The listing builds one solid part. Answer for the finished solid, in the listing's coordinates (mm). Round coordinates to 2 decimals unless told otherwise and drop trailing zeros. Order: outer loops, then holes, each group sorted by start corner. A loop starts at its lowest first (then second) coordinate and runs counter-clockwise, first axis right, second up. Notation, with made-up numbers: (16, -26.75) -> (41, -26.75) arc R16 cw to (41, -4.75) -> close; hole circle Ø10 at (83, 34). An arc over 180 degrees is marked (long way). Return JSON: item names as keys, results as strings. Group by question number.
(1) Each of these flat-tipped pins is pushed along its axis until it touches: pin 1 (1.5 mm diameter, centred on x = 1.5, z = 49, fed in from -Y); pin 2 (1.4 mm diameter, centred on x = 1, z = 58, fed in from +Y). Where does it stop, or does it pass through?
(2) The part is cut by section C-C (z = 31). Determine the outline of the cut face in (x, y), plus the area to 3 significant figures.
(3) The part is cut by section A-A (x = 2.1). Determine the outline of the cut face in (y, z) (1 decimal).
(4) The part is cut by section D-D (y = 71.5). Determine the outline of the cut face in (x, z).
(5) Consider line 1 (Z direction, x = 2.8, y = 44); line 2 (Z direction, x = 0.2, y = 46.5); line 3 (Y direction, x = 2.4, z = 66.5). Determine where each line is inside the solid, lowest interval first. Write a range as [from, to].
(6) The part is cut by section B-B (y = 50). Determine the outline of the cut face in (x, z), plus the area to 3 significant figures.
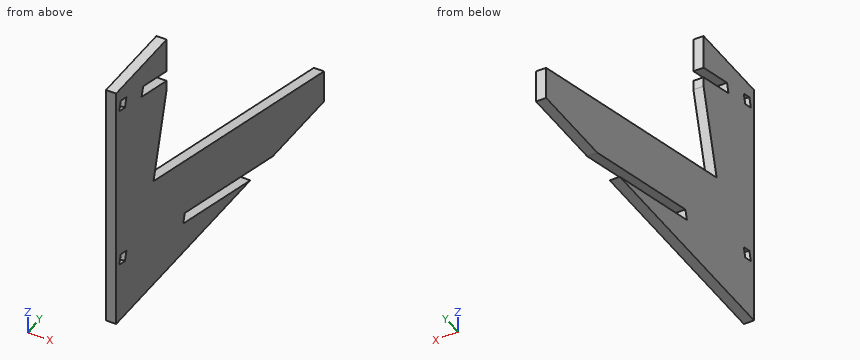
from build123d import *

# Parameters (mm, degrees)
BOSS_EXTRUDE1_DEPTH = 2.93
CUT_EXTRUDE4_DEPTH  = 3.93
CUT_EXTRUDE6_DEPTH  = 3.93
CUT_EXTRUDE7_DEPTH  = 3.93
CUT_EXTRUDE9_DEPTH  = 3.93


with BuildPart() as part:
    # Sketch1 → Boss-Extrude1 (new body)
    with BuildSketch(Plane(origin=(0, 0, 0), x_dir=(0, 0, -1), z_dir=(1, 0, 0))):
        Polygon((0, 0), (0, 104.696802211), (-9.525, 104.696802211), (-32.53401311, 18.825996254), (-57.068529097, 25.4), (-72.943529097, 25.4), (-72.943529097, 0), align=None)
    extrude(amount=BOSS_EXTRUDE1_DEPTH)

    # Sketch5 → Cut-Extrude4 (cut, through all)
    with BuildSketch(Plane(origin=(2.93, 0, 0), x_dir=(0, 0, -1), z_dir=(1, 0, 0))):
        Polygon((0, 67.5876455), (0, 78.908296184), (-11.885190186, 34.552162552), (-9.055027515, 33.79382275), align=None)
    extrude(amount=-CUT_EXTRUDE4_DEPTH, mode=Mode.SUBTRACT)

    # Sketch7 → Cut-Extrude6 (cut, through all)
    with BuildSketch(Plane.ZY):
        Polygon((63.256615243, 12.832490583), (66.086777914, 13.590830386), (62.719323915, 26.158339802), (59.889161244, 25.4), align=None)
    extrude(amount=-CUT_EXTRUDE6_DEPTH, mode=Mode.SUBTRACT)

    # Sketch9 → Cut-Extrude7 (cut, through all)
    with BuildSketch(Plane.ZY):
        Polygon((65.511361587, 4.417662671), (68.341524258, 5.176002473), (69.09986406, 2.345839802), (66.269701389, 1.5875), align=None)
    extrude(amount=-CUT_EXTRUDE7_DEPTH, mode=Mode.SUBTRACT)

    # Sketch11 → Cut-Extrude9 (cut, through all)
    with BuildSketch(Plane.ZY):
        Polygon((17.683407431, 1.592270516), (20.513570102, 2.350610318), (19.7552303, 5.180772989), (16.925067629, 4.422433187), align=None)
    extrude(amount=-CUT_EXTRUDE9_DEPTH, mode=Mode.SUBTRACT)


solid = part.part
Answer below:
{
 "1": {"pin 1": "stops at y = 0", "pin 2": "stops at y = 25.4"},
 "2": {"outline": "(0, 0) -> (2.93, 0) -> (2.93, 24.55) -> (0, 24.55) -> close", "area": "71.9 mm²"},
 "3": {"outline": "(0, 0) -> (67.6, 0) -> (33.8, 9.1) -> (34.6, 11.9) -> (78.9, 0) -> (104.7, 0) -> (104.7, 9.5) -> (18.8, 32.5) -> (25.4, 57.1) -> (25.4, 59.9) -> (12.8, 63.3) -> (13.6, 66.1) -> (25.4, 62.9) -> (25.4, 72.9) -> (0, 72.9) -> close; hole (1.6, 17.7) -> (4.4, 16.9) -> (5.2, 19.8) -> (2.4, 20.5) -> close; hole (1.6, 66.3) -> (4.4, 65.5) -> (5.2, 68.3) -> (2.3, 69.1) -> close"},
 "4": {"outline": "(0, 1.99) -> (2.93, 1.99) -> (2.93, 18.42) -> (0, 18.42) -> close"},
 "5": {"line 1": "z = [0, 6.32], [9.35, 25.79]", "line 2": "z = [0, 5.65], [8.68, 25.12]", "line 3": "y = [0, 1.65], [4.68, 25.4]"},
 "6": {"outline": "(0, 0) -> (2.93, 0) -> (2.93, 4.71) -> (0, 4.71) -> close; (0, 7.75) -> (2.93, 7.75) -> (2.93, 24.18) -> (0, 24.18) -> close", "area": "62.0 mm²"}
}
